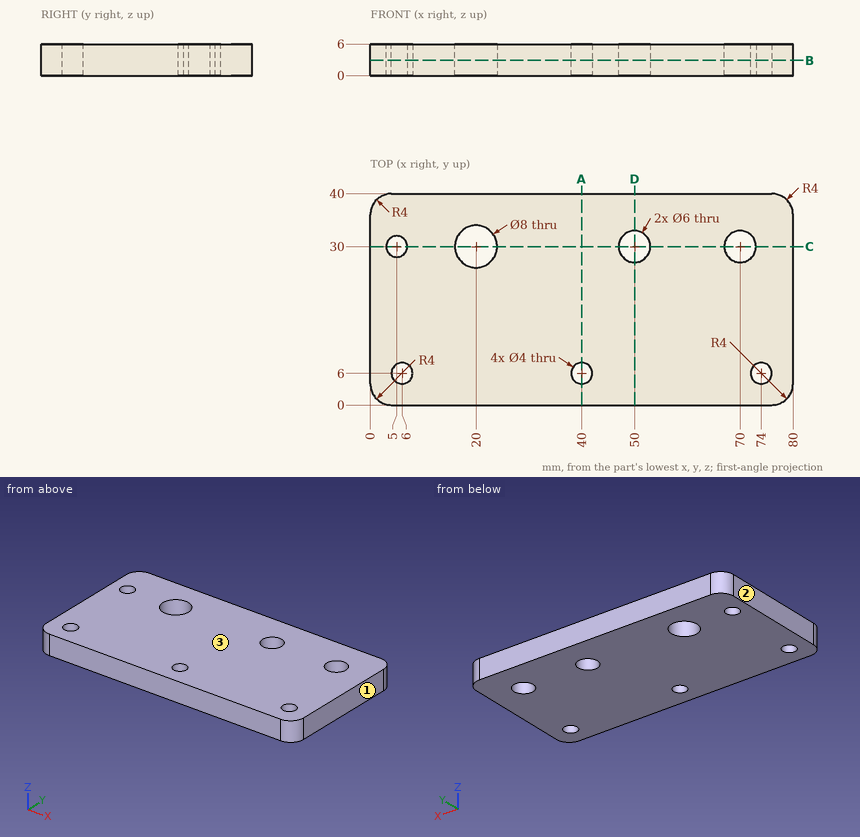
Can you work these out from the drawing? Everything is in mm from the part's minimum corner. Round coordinates to 2 decimals unless told otherwise and drop trailing zeros. Order: outer loops, then holes, each group sorted by start corner. A loop starts at its lowest first (then second) coordinate and runs counter-clockwise, first axis right, second up. Notation, with made-up numbers: (18, 62.5) - (47, 62.5) arc R22 cw to (47, 73.5) - close; hole circle Ø10 at (-36.5, 53). An arc over 180 degrees is marked (long way). Answer in a Markdown table with one row per item.
(1) Suppose I cut it at D-D, the plane x = 50. Please give me the cut outline in (y, z).
From the geometry:
| item | result |
|---|---|
| outline | (0, 0) - (27, 0) - (27, 6) - (0, 6) - close; (33, 0) - (40, 0) - (40, 6) - (33, 6) - close |
(2) Suppose I cut it at C-C, the plane y = 30. Please give me the cut outline in (x, z).
From the geometry:
| item | result |
|---|---|
| outline | (0, 0) - (3, 0) - (3, 6) - (0, 6) - close; (7, 0) - (16, 0) - (16, 6) - (7, 6) - close; (24, 0) - (47, 0) - (47, 6) - (24, 6) - close; (53, 0) - (67, 0) - (67, 6) - (53, 6) - close; (73, 0) - (80, 0) - (80, 6) - (73, 6) - close |
(3) Suppose I cut it at A-A, the plane x = 40. Please give me the cut outline in (y, z).
From the geometry:
| item | result |
|---|---|
| outline | (0, 0) - (4, 0) - (4, 6) - (0, 6) - close; (8, 0) - (40, 0) - (40, 6) - (8, 6) - close |
(4) Suppose I cut it at B-B, the plane z = 2.9. Please give me the cut outline in (x, y).
From the geometry:
| item | result |
|---|---|
| outline | (0, 4) arc R4 ccw to (4, 0) - (76, 0) arc R4 ccw to (80, 4) - (80, 36) arc R4 ccw to (76, 40) - (4, 40) arc R4 ccw to (0, 36) - close; hole circle Ø4 at (5, 30); hole circle Ø4 at (6, 6); hole circle Ø8 at (20, 30); hole circle Ø4 at (40, 6); hole circle Ø6 at (50, 30); hole circle Ø6 at (70, 30); hole circle Ø4 at (74, 6) |
(5) If we mould it in two halves opening along X, with no side actions, what happens to the marked faces 1, 2 and 3? For each: released by +X, released by -X, zero draft, split by the parting line, or undercut.
From the geometry:
| item | result |
|---|---|
| face 1 | released by +X |
| face 2 | released by -X |
| face 3 | zero draft |
(6) Please list where these lines run through material, in increasing order: L1, parallel to Y at x = 74, z = 1.5; L2, parallel to X at y = 4.5, z = 1.6; L3, parallel to Y at x = 75.5, z = 4.1. Write a range as from..to.
From the geometry:
| item | result |
|---|---|
| L1 | y = 0..4, 8..40 |
| L2 | x = 0..4.68, 7.32..38.68, 41.32..72.68, 75.32..80 |
| L3 | y = 0..4.68, 7.32..40 |
(7) For P1, Ø3, axis at x = 40, y = 6, coming from the -Z side, with a flat end and sliding along its axis, tell me the tip position at first contact or that it passes through.
From the geometry:
| item | result |
|---|---|
| P1 | passes through |
